Check sheet for the modelled part. Datum: model origin and axes. Units: mm. Face numbers are marked on the shaded views. A direction names the side the tool comes from. Round coordinates to 2 decimals unless told otherwise and drop trailing zeros. Loops run counter-clockwise (first coordinate to the right, second up) from the corner with the lowest first, then second, coordinate; pieces in that order, holes last. Notation, with made-up numbers: (14, 79.5) - (41, 79.5) arc R22 ccw to (41, 107.5) - close; hole circle Ø1 at (25, 6.25). An arc over 180 degrees is marked (long way). Put each result on its own line as item: value. Start each with the question number.
```python
from build123d import *

# Parameters (mm, degrees)
BOSS_EXTRUDE1_DEPTH = 34.8
CUT_EXTRUDE1_REACH  = 68.182
SKETCH2_R           = 1.7
SKETCH3_R           = 0.8
CUT_EXTRUDE2_DEPTH  = 6
SKETCH4_R           = 1.25
CUT_EXTRUDE3_DEPTH  = 10
SKETCH5_R           = 1
CUT_EXTRUDE4_DEPTH  = 4
SKETCH6_R           = 3.25
CUT_EXTRUDE5_DEPTH  = 3


with BuildPart() as part:
    # Sketch1 → Boss-Extrude1 (new body)
    with BuildSketch(Plane.XY):
        Polygon((0, 0), (27, 0), (27, -5), (33, -5), (33, 2), (55, 2), (55, 7), (0, 7), align=None)
    extrude(amount=-BOSS_EXTRUDE1_DEPTH)

    # Sketch2 → Cut-Extrude1 (cut, up to next)
    with BuildSketch(Plane(origin=(0, 7, 0), x_dir=(1, 0, 0), z_dir=(0, 1, 0)), mode=Mode.PRIVATE) as cut_extrude1_sk1:
        with Locations(Location((3.5, 24.9, 0), (0, 0, 180))):
            Circle(SKETCH2_R)
    cut_extrude1_tool1 = extrude(cut_extrude1_sk1.sketch, amount=-CUT_EXTRUDE1_REACH, mode=Mode.PRIVATE) & part.part
    # Sketch2 → Cut-Extrude1 (cut, up to next)
    with BuildSketch(Plane(origin=(0, 7, 0), x_dir=(1, 0, 0), z_dir=(0, 1, 0)), mode=Mode.PRIVATE) as cut_extrude1_sk2:
        with Locations(Location((23.5, 24.9, 0), (0, 0, 180))):
            Circle(SKETCH2_R)
    cut_extrude1_tool2 = extrude(cut_extrude1_sk2.sketch, amount=-CUT_EXTRUDE1_REACH, mode=Mode.PRIVATE) & part.part
    # Sketch2 → Cut-Extrude1 (cut, up to next)
    with BuildSketch(Plane(origin=(0, 7, 0), x_dir=(1, 0, 0), z_dir=(0, 1, 0)), mode=Mode.PRIVATE) as cut_extrude1_sk3:
        with Locations(Location((23.5, 9.9, 0), (0, 0, 180))):
            Circle(SKETCH2_R)
    cut_extrude1_tool3 = extrude(cut_extrude1_sk3.sketch, amount=-CUT_EXTRUDE1_REACH, mode=Mode.PRIVATE) & part.part
    # Sketch2 → Cut-Extrude1 (cut, up to next)
    with BuildSketch(Plane(origin=(0, 7, 0), x_dir=(1, 0, 0), z_dir=(0, 1, 0)), mode=Mode.PRIVATE) as cut_extrude1_sk4:
        with Locations(Location((3.5, 9.9, 0), (0, 0, 180))):
            Circle(SKETCH2_R)
    cut_extrude1_tool4 = extrude(cut_extrude1_sk4.sketch, amount=-CUT_EXTRUDE1_REACH, mode=Mode.PRIVATE) & part.part
    add(cut_extrude1_tool1.solids().sort_by_distance((3.5, 7, -24.9))[0], mode=Mode.SUBTRACT)
    add(cut_extrude1_tool2.solids().sort_by_distance((23.5, 7, -24.9))[0], mode=Mode.SUBTRACT)
    add(cut_extrude1_tool3.solids().sort_by_distance((23.5, 7, -9.9))[0], mode=Mode.SUBTRACT)
    add(cut_extrude1_tool4.solids().sort_by_distance((3.5, 7, -9.9))[0], mode=Mode.SUBTRACT)

    # Sketch3 → Cut-Extrude2 (cut)
    with BuildSketch(Plane(origin=(33, 0, 0), x_dir=(0, 0, -1), z_dir=(1, 0, 0))):
        with Locations((8.9, -1)):
            Circle(SKETCH3_R)
        with Locations(Location((25.9, -1, 0), (0, 0, 180))):
            Circle(SKETCH3_R)
    extrude(amount=-CUT_EXTRUDE2_DEPTH, mode=Mode.SUBTRACT)

    # Sketch4 → Cut-Extrude3 (cut)
    with BuildSketch(Plane(origin=(55, 0, 0), x_dir=(0, 0, -1), z_dir=(1, 0, 0))):
        with Locations((4.4, 4.5)):
            Circle(SKETCH4_R)
        with Locations(Location((30.4, 4.5, 0), (0, 0, 180))):
            Circle(SKETCH4_R)
    extrude(amount=-CUT_EXTRUDE3_DEPTH, mode=Mode.SUBTRACT)

    # Sketch5 → Cut-Extrude4 (cut)
    with BuildSketch(Plane(origin=(55, 0, 0), x_dir=(0, 0, -1), z_dir=(1, 0, 0))):
        with Locations((10.4, 4.5)):
            Circle(SKETCH5_R)
        with Locations(Location((24.4, 4.5, 0), (0, 0, 180))):
            Circle(SKETCH5_R)
    extrude(amount=-CUT_EXTRUDE4_DEPTH, mode=Mode.SUBTRACT)

    # Sketch6 → Cut-Extrude5 (cut)
    with BuildSketch(Plane(origin=(0, 7, 0), x_dir=(1, 0, 0), z_dir=(0, 1, 0))):
        with Locations(Location((3.5, 24.9, 0), (0, 0, 180))):
            Circle(SKETCH6_R)
        with Locations(Location((23.5, 24.9, 0), (0, 0, 180))):
            Circle(SKETCH6_R)
        with Locations(Location((23.5, 9.9, 0), (0, 0, 180))):
            Circle(SKETCH6_R)
        with Locations(Location((3.5, 9.9, 0), (0, 0, 180))):
            Circle(SKETCH6_R)
    extrude(amount=-CUT_EXTRUDE5_DEPTH, mode=Mode.SUBTRACT)


solid = part.part
```
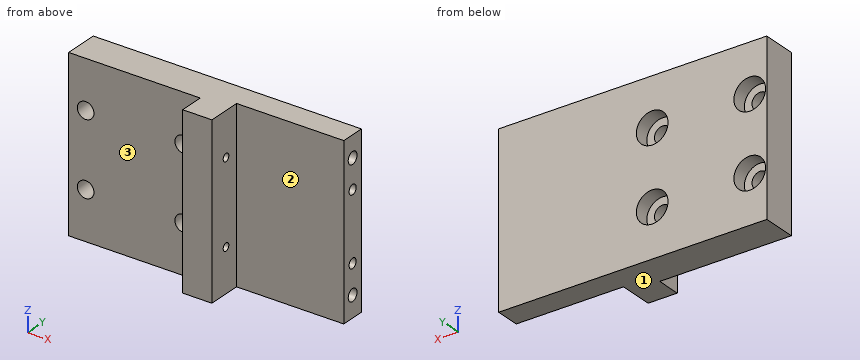
Q1. Cross-section at B-B on z = -30.4. Enter the section's corners in (x, y).
Q2. Depth check by flat-ended pin: pin 1 Ø4 at (x, z) = (23.5, -9.9) entering from -Y; pin 2 Ø17.5 at (x, z) = (43.5, -23) entering from -Y; pin 3 Ø6 at (x, z) = (3.5, -24.9) entering from +Y. Enter the tip coordinate at first touch or a pass-through.
Q3. Cross-section at D-D on x = 39.5. Enter the section's corners in (y, z), and give its area (3 significant figures).
Q4. Cross-section at A-A on y = -1. Enter the section's corners in (x, z).
Q5. Material ranges on line 1 (Z direction, x = 3.5, y = 2.5); line 2 (Z direction, x = 3.5, y = 5.15); line 3 (Y direction, x = 51.5, z = -30.4), recorded low to high. Write a range as from..to.
Q6. Cross-section at C-C on x = 24.5. Enter the section's corners in (y, z).
Q7. Set-up check for the marked faces 1, 2 and 3: record each of +Z, -Z, +X, -X, +Y, -Y from which the full face is reachable in a straight line by a thin tool's end or side.
Answer list:
1. outline: (0, 0) - (27, 0) - (27, -5) - (33, -5) - (33, 2) - (55, 2) - (55, 3.25) - (45, 3.25) - (45, 5.75) - (55, 5.75) - (55, 7) - (0, 7) - close
2. pin 1: stops at y = 0
2. pin 2: stops at y = 2
2. pin 3: stops at y = 4
3. outline: (2, -34.8) - (7, -34.8) - (7, 0) - (2, 0) - close
3. area: 174 mm2
4. outline: (27, -34.8) - (33, -34.8) - (33, -26.7) - (27, -26.7) - close; (27, -25.1) - (33, -25.1) - (33, -9.7) - (27, -9.7) - close; (27, -8.1) - (33, -8.1) - (33, 0) - (27, 0) - close
5. line 1: z = -34.8..-26.6, -23.2..-11.6, -8.2..0
5. line 2: z = -34.8..-28.15, -21.65..-13.15, -6.65..0
5. line 3: y = 2..3.25, 5.75..7
6. outline: (0, -34.8) - (7, -34.8) - (7, -27.99) - (4, -27.99) - (4, -26.27) - (0, -26.27) - close; (0, -23.53) - (4, -23.53) - (4, -21.81) - (7, -21.81) - (7, -12.99) - (4, -12.99) - (4, -11.27) - (0, -11.27) - close; (0, -8.53) - (4, -8.53) - (4, -6.81) - (7, -6.81) - (7, 0) - (0, 0) - close
7. face 1: -Z, +X, -X, +Y, -Y
7. face 2: +Z, -Z, +X, -Y
7. face 3: +Z, -Z, -X, -Y
